from build123d import *

# Parameters (mm, degrees)
F2_W     = 6.9
F2_H     = 4.8
F3_DEPTH = 2
F4_R     = 2.1
F5_SIZE  = 0.2
F6_R     = 1.1


# Not quite as in the source:
# - a feature names something its author has since deleted; it is built from what else it names


with BuildPart() as f1:
    # F0 (on Front) → F1 (revolve)
    with BuildSketch(Plane.XZ):
        Polygon((3.1, 0), (3.1, -12.1), (5.95, -12.1), (5.95, -2), (7.9, -2), (7.9, 0), (5.95, 0), (5.95, 8), (3.1, 8), align=None)
    revolve(axis=Axis((0, 0, -6.05), (0, 0, -1)))

    # F2 (on face) → F3 (join)
    with BuildSketch(Plane.XY):
        with Locations((6.55, 0)):
            Rectangle(F2_W, F2_H)
        with Locations((-6.55, 0)):
            Rectangle(F2_W, F2_H)
    extrude(amount=-F3_DEPTH)

    # F4
    f4_edges = [f1.edges().sort_by_distance(p)[0] for p in [
        (7.526619, -2.4, -1),
        (7.526619, 2.4, -1),
        (-7.526619, 2.4, -1),
        (-7.526619, -2.4, -1),
    ]]
    fillet(f4_edges, radius=F4_R)

    # F5
    f5_edges = [f1.edges().sort_by_distance(p)[0] for p in [
        (3.1, 0, -2.05),
        (-3.1, 0, -12.1),
        (-3.1, 0, 8),
        (-3.1, 0, -1),
        (10, -2.4, -1),
        (10, 2.4, -1),
        (10, 0, 0),
        (10, 0, -2),
        (0, -7.9, -2),
        (0, -7.9, 0),
        (9.465143, -2.4, 0),
        (9.465143, -2.4, -2),
        (9.465143, 2.4, 0),
        (9.465143, 2.4, -2),
        (-10, 2.4, -1),
        (-10, -2.4, -1),
        (-10, 0, 0),
        (-10, 0, -2),
        (-9.465143, -2.4, 0),
        (-9.465143, -2.4, -2),
        (-9.465143, 2.4, -2),
        (-9.465143, 2.4, 0),
        (-5.95, 0, 8),
        (-5.95, 0, -12.1),
        (7.829036, -2.711914, 0),
        (-7.829036, -2.711914, 0),
        (7.829036, 2.711914, 0),
        (0, 7.9, 0),
        (-7.829036, 2.711914, 0),
        (7.829036, -2.711914, -2),
        (-7.829036, -2.711914, -2),
        (7.829036, 2.711914, -2),
        (0, 7.9, -2),
        (-7.829036, 2.711914, -2),
    ]]
    chamfer(f5_edges, length=F5_SIZE)

    # F6
    f6_edges = [f1.edges().sort_by_distance(p)[0] for p in [
        (-5.95, 0, -2),
        (-5.95, 0, 0),
    ]]
    fillet(f6_edges, radius=F6_R)


solid = f1.part
Verification items for the finished model (mm, model axes). A direction names the side the tool comes from. Round coordinates to 2 decimals unless told otherwise and drop trailing zeros. Order: outer loops, then holes, each group sorted by start corner. A loop starts at its lowest first (then second) coordinate and runs counter-clockwise, first axis right, second up. Notation, with made-up numbers: (-32.5, 15) -> (-7.5, 15) arc R19 ccw to (-7.5, 34) -> close; hole circle Ø5 at (31.5, 77.25). An arc over 180 degrees is marked (long way). Put each result on its own line as item: value.
1) Set-up check for faces 5 (the flat face through (10, 0, -1)), 6 (the cylindrical face through (-4.385, -4.021, 4.497)), 7 (the cylindrical face through (-4.385, -4.021, -7.438)), 8 (the flat face through (9.4, -2.4, -1)), 9 (the flat face through (-9.4, 2.4, -1)): record each of +Z, -Z, +X, -X, +Y, -Y from which the full face is reachable in a straight line by a thin tool's end or side.
Final values:
face 5: +Z, -Z, +X, +Y, -Y
face 6: +Z
face 7: -Z
face 8: +Z, -Z, +X, -Y
face 9: +Z, -Z, -X, +Y
2) Mould release check, pull along Y, two halves, no side actions. Record for faces 1 (the flat face through (9.4, 2.4, -1)), 2 (the flat face through (-10, 0, -1)), 3 (the cylindrical face through (1.43, 2.75, -2.19)), 4 (the cylindrical face through (7.815, -2.72, -0.989)): +Y half, -Y half, draft (parallel to the pull), parting line (faces both ways), or undercut.
Final values:
face 1: +Y half
face 2: draft
face 3: undercut
face 4: -Y half
3) Material ranges on line 1 (Y direction, x = 0, z = -3.5); line 2 (Z direction, x = -5.5, y = -4.5), recorded low to high.
Final values:
line 1: y = -5.95 to -3.1, 3.1 to 5.95
line 2: z = -2 to 0
4) Section check C-C (z = 2). Record the cut outline in (x, y), then the cut area to 3 significant figures.
Final values:
outline: circle Ø11.9 at (0, 0); hole circle Ø6.2 at (0, 0)
area: 81.0 mm^2
5) Depth check by flat-ended pin: pin 1 (2 mm diameter, centred on x = 0, z = -6.5, fed in from +Y); pin 2 (3 mm diameter, centred on y = 6, z = 5.5, fed in from -X); pin 3 (0.7 mm diameter, centred on x = -9, z = -1, fed in from -Y); pin 4 (5 mm diameter, centred on x = 0, y = 0, fed in from -Z). Enter the tip coordinate at first touch or a pass-through.
Final values:
pin 1: stops at y = 5.95
pin 2: stops at x = -3.89
pin 3: stops at y = -2.42
pin 4: passes through
